Part model, mm, in its own coordinate system. A direction names the side the tool comes from. Coordinates: 2 decimals unless noted, no trailing zeros. Loops run counter-clockwise (first coordinate to the right, second up) from the corner with the lowest first, then second, coordinate; pieces in that order, holes last. Notation, with made-up numbers: (-4.5, -39) -> (53.5, -39) arc R16 cw to (53.5, -33) -> close; hole circle Ø9 at (-30, -29.5). An arc over 180 degrees is marked (long way). One line per item, written item: value. Start each with the question number.
from build123d import *

# Parameters (mm, degrees)
SWEEP1_PROFILE_R    = 10
SWEEP2_PROFILE_R    = 10
SHELL2_START        = -57.391158908
SHELL2_OUTLINE_R    = 8
SHELL2_DEPTH        = 120
SHELL2_START_2      = -1e-07
SHELL2_2_OUTLINE_R  = 8
SHELL2_2_DEPTH      = 69.282032403
SKETCH27_R          = 11.5
BOSS_EXTRUDE2_DEPTH = 3
SCALE1_SCALE        = 0.1


with BuildPart() as part:
    # Sweep1: sweep along a path in Sketch3
    with BuildLine(Plane.XY) as sweep1_path:
        Line((-57.391158908, 0), (62.608841092, 0))
    # Sweep1 profile (on start of the path) → Sweep1 (sweep)
    with BuildSketch(Plane(origin=(-57.391158908, 0, 0), x_dir=(0, 0, 1), z_dir=(1, 0, 0))):
        Circle(SWEEP1_PROFILE_R)
    sweep(path=sweep1_path.line)

    # Sweep2: sweep along a path in Sketch3<4>
    with BuildLine(Plane.XY) as sweep2_path:
        Line((0, 0), (60, -34.641016151))
    # Sweep2 profile (on start of the path) → Sweep2 (sweep)
    with BuildSketch(Plane(origin=(0, 0, 0), x_dir=(0.500000000000001, 0.8660254037844382, 0), z_dir=(0.8660254037844382, -0.500000000000001, 0))):
        Circle(SWEEP2_PROFILE_R)
    sweep(path=sweep2_path.line)

    # Shell2: read off the stored shape, not the designer's step
    # Shell2 outline → Shell2 (cut)
    with BuildSketch(Plane.YZ.offset(SHELL2_START)):
        Circle(SHELL2_OUTLINE_R)
    extrude(amount=SHELL2_DEPTH, mode=Mode.SUBTRACT)

    # Shell2 2 outline → Shell2 2 (cut)
    with BuildSketch(Plane(origin=(0, 0, 0), x_dir=(0.500000000000001, 0.866025403784438, 0), z_dir=(0.866025403784438, -0.500000000000001, 0)).offset(SHELL2_START_2)):
        Circle(SHELL2_2_OUTLINE_R)
    extrude(amount=SHELL2_2_DEPTH, mode=Mode.SUBTRACT)

    # Sketch27 → Boss-Extrude2 (add)
    with BuildSketch(Plane(origin=(62.608841092, 0, 0), x_dir=(0, 0, -1), z_dir=(1, 0, 0))):
        Circle(SKETCH27_R)
    extrude(amount=BOSS_EXTRUDE2_DEPTH)


with BuildPart() as part_1:
    # Scale1: scaled about (0, 0, 0)
    add(part.part.scale(SCALE1_SCALE))


solid = part_1.part
1) Pull direction X, two halves, no side cores. Call faces 1 (the cylindrical face through (0, 1, 0)), 2 (the flat face through (6.561, 0, 0)): +X half, -X half, draft (parallel to the pull), parting line (faces both ways), or undercut.
2) Slice it at C-C (y = 0.4). Give the cut face in (x, z).
3) Tool access for faces 3 (the cylindrical face through (0.177, 0.763, 0.24)), 4 (the cylindrical face through (3.2, -3, 0)): list every direction of +Z, -Z, +X, -X, +Y, -Y with a clear straight run to the whole face (end or side of a thin tool).
4) Probe line 1 (Z direction, x = 3, y = -1.8); line 2 (Y direction, x = 5, z = 0.25); line 3 (X direction, y = -0.2, z = 0). List the from-to ranges inside material, lowest first. Write a range as from..to.
5) Pin check, flat tips, straight feed: pin 1 Ø2 at (x, y) = (-1.5, -1) entering from -Z; pin 2 Ø3 at (x, y) = (-4, -3.5) entering from +Z; pin 3 Ø1.5 at (x, y) = (1, -1.5) entering from +Z; pin 4 Ø1 at (y, z) = (0, 0) entering from -X. Stop position of each tip, or through.
6) Slice it at A-A (z = 0.2). Give the cut face in (x, y), then the cut area to 3 significant figures.
7) Slice it at B-B (x = -4.5). Give the cut face in (y, z).
Check sheet entries:
1. face 1: undercut
1. face 2: +X half
2. outline: (-5.74, -0.92) -> (6.26, -0.92) -> (6.26, -1.08) -> (6.56, -1.08) -> (6.56, 1.08) -> (6.26, 1.08) -> (6.26, 0.92) -> (-5.74, 0.92) -> (-5.74, 0.69) -> (6.26, 0.69) -> (6.26, -0.69) -> (-5.74, -0.69) -> close
3. face 3: -X
3. face 4: none
4. line 1: z = -1..-0.8, 0.8..1
4. line 2: y = -4..-3.76, -2.01..-1.77, -0.97..-0.76, 0.76..0.97
4. line 3: x = 6.26..6.56
5. pin 1: stops at z = -1
5. pin 2: passes through
5. pin 3: stops at z = 1
5. pin 4: stops at x = 6.26
6. outline: (-5.74, -0.98) -> (-0.26, -0.98) -> (5.51, -4.31) -> (5.61, -4.13) -> (-0.21, -0.77) -> (-5.74, -0.77) -> close; (-5.74, 0.77) -> (6.26, 0.77) -> (6.26, -0.77) -> (2.89, -0.77) -> (6.39, -2.79) -> (6.49, -2.62) -> (3.66, -0.98) -> (6.26, -0.98) -> (6.26, -1.13) -> (6.56, -1.13) -> (6.56, 1.13) -> (6.26, 1.13) -> (6.26, 0.98) -> (-5.74, 0.98) -> close
6. area: 7.01 mm^2
7. outline: circle Ø2 at (0, 0); hole circle Ø1.6 at (0, 0)
